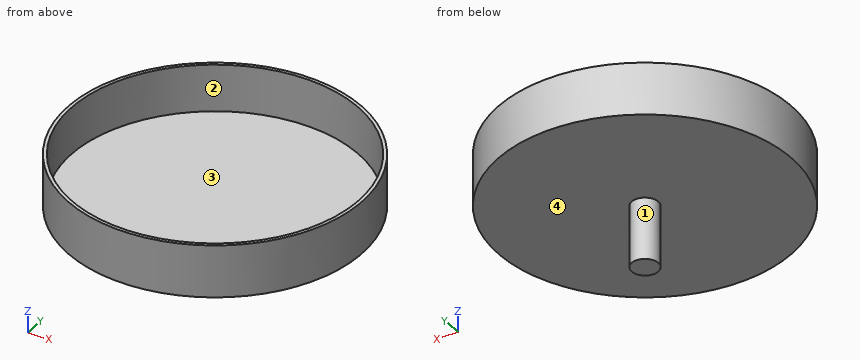
from build123d import *

# Parameters (mm, degrees)
SKETCH1_R      = 21.9
EXTRUDE1_DEPTH = 0.8
SKETCH2_R      = 21.9
SKETCH2_R_2    = 21.4
EXTRUDE2_DEPTH = 7
SKETCH4_R      = 2
EXTRUDE4_DEPTH = 10


with BuildPart() as part:
    # Sketch1 → Extrude1 (new body)
    with BuildSketch(Plane.XY):
        Circle(SKETCH1_R)
    extrude(amount=EXTRUDE1_DEPTH)

    # Sketch2 → Extrude2 (add)
    with BuildSketch(Plane.XY.offset(0.8)):
        Circle(SKETCH2_R)
        Circle(SKETCH2_R_2, mode=Mode.SUBTRACT)
    extrude(amount=EXTRUDE2_DEPTH)

    # Sketch4 → Extrude4 (add)
    with BuildSketch(Plane.XY.offset(0.8)):
        Circle(SKETCH4_R)
    extrude(amount=-EXTRUDE4_DEPTH)


solid = part.part
Geometry check sheet. Reference: the model listing, model coordinates, mm. Face numbers are marked on the shaded views. Round coordinates to 2 decimals unless told otherwise and drop trailing zeros. Loops run counter-clockwise (first coordinate to the right, second up) from the corner with the lowest first, then second, coordinate; pieces in that order, holes last.
Item 1: Cross-section at C-C on z = 3. Record the boundary of the cut face in (x, y), then the cut area to 3 significant figures.
Item 2: Cross-section at A-A on x = 0. Record the boundary of the cut face in (y, z).
Item 3: Mould release check, pull along X, two halves, no side actions. Record for the marked faces 1, 2, 3 and 4: pulls with the +X half, pulls with the -X half, needs draft (parallel to the pull), parting line crosses it, or undercut.
Item 4: Cross-section at D-D on z = -7.5. Record the boundary of the cut face in (x, y).
Item 5: Gauge pin test, flat ends, axial feed: pin 1 (21.5 mm diameter, centred on x = -8.5, y = 5, fed in from +Z); pin 2 (1.5 mm diameter, centred on y = 17.5, z = 4, fed in from -X); pin 3 (1 mm diameter, centred on y = -14, z = 3, fed in from +X). Record the tip position at first contact, or that the pin passes through.
Item 6: Thickness scan on line 1 (Y direction, x = 0, z = 5.75); line 2 (Z direction, x = 15, y = -12); line 3 (X direction, y = 13, z = 5). Record the ranges inside material, lowest first.
Answer sheet:
1. outline: circle Ø43.8 at (0, 0); hole circle Ø42.8 at (0, 0)
1. area: 68.0 mm2
2. outline: (-21.9, 0) - (-2, 0) - (-2, -9.2) - (2, -9.2) - (2, 0) - (21.9, 0) - (21.9, 7.8) - (21.4, 7.8) - (21.4, 0.8) - (-21.4, 0.8) - (-21.4, 7.8) - (-21.9, 7.8) - close
3. face 1: parting line crosses it
3. face 2: undercut
3. face 3: undercut
3. face 4: needs draft
4. outline: circle Ø4 at (0, 0)
5. pin 1: stops at z = 0.8
5. pin 2: stops at x = -14.11
5. pin 3: stops at x = 17.24
6. line 1: y = -21.9 to -21.4, 21.4 to 21.9
6. line 2: z = 0 to 0.8
6. line 3: x = -17.62 to -17, 17 to 17.62
